The listing builds one solid part. Answer for the finished solid, in the listing's coordinates (mm). A direction names the side the tool comes from. Round coordinates to 2 decimals unless told otherwise and drop trailing zeros. Write each loop counter-clockwise with the first axis right and the second up, starting at its lowest first coordinate (ties: lowest second). Pieces come first, ordered by that corner, then holes. Notation, with made-up numbers: (67.25, -18) -> (97.25, -18) arc R16 ccw to (97.25, 9) -> close; hole circle Ø5 at (57, 84). An arc over 180 degrees is marked (long way). Write each question's results on one line, items separated by ' | '. Start each with the question number.
Autodesk Fusion 360 part; units mm, degrees
sketch "Sketch1" plane through (0, 0, 0) normal (0, 1, 0) x (1, 0, 0)
  line L0 (0, 0) -> (4, 0)
  line L1 (4, 0) -> (4, -4)
  line L2 (4, -4) -> (0, -4)
  line L3 (0, -4) -> (0, 0)
  circle A0 centre (2, -2) radius 0.8
  dimension "d1" = 4
  dimension "d2" = 4
  dimension "d3" = 1.6
  dimension "d4" = 2
  dimension "d5" = 2
extrude "Extrude1" add sketch "Sketch1" along normal blind 14 makes body 1
sketch "Sketch2" plane through (0, 0, 4) normal (0, 0, 1) x (-1, 0, 0)
  line L0 (0, 0) -> (-4, 0)
  line L1 (-4, 0) -> (-4, -14)
  line L2 (-4, -14) -> (0, -14)
  line L3 (0, -14) -> (0, 0)
  line L4 (-4, -14) -> (0, -14)
  line L5 (0, -14) -> (0, -10)
  line L6 (0, -10) -> (-4, -10)
  line L7 (-4, -10) -> (-4, -14)
  circle A0 centre (-2, -12) radius 0.8
  dimension "d8" = 4
  dimension "d9" = 1.6
  dimension "d10" = 2
  dimension "d11" = 2
extrude "Extrude2" add sketch "Sketch2" along normal blind 10 contours L1 L2 L3 L4 L5 L6 L7 bodies 1
ref_plane "WorkPlane1" through (4, 7, 0) normal (0.9397, 0, -0.342) x (0, 1, 0)
sketch "Sketch3" plane through (4, 7, 0) normal (0.9397, 0, -0.342) x (0, 1, 0)
  line L0 (-7, 3.7588) -> (-7, 0)
  line L1 (-7, 0) -> (7, 0)
  line L2 (7, 0) -> (7, 13.1557)
  line L3 (7, 13.1557) -> (3, 13.1557)
  line L4 (3, 13.1557) -> (3, 3.7588)
  line L5 (3, 3.7588) -> (-7, 3.7588)
  line L6 (7, 0) -> (3, 0)
  line L7 (3, 0) -> (3, 3.7588)
  line L8 (3, 3.7588) -> (7, 3.7588)
  line L9 (7, 3.7588) -> (7, 0)
  circle A0 centre (5, 1.7588) radius 0.8
  dimension "d15" = 1.6
  dimension "d16" = 2
  dimension "d17" = 2
extrude "Extrude3" add sketch "Sketch3" along normal blind 10 separate body contours L1 L2 L6 L7 L8 L9 makes body 2
extrude "Extrude4" add 1 faces at (5.1485, 12.0199, 3.1555) along direction (-0.939693, 0, 0.34202) up to surface end surface through (4, 0, 0) normal (1, 0, 0) offset 0 on bodies 2 bodies 2 1
extrude "Extrude5" add sketch "Sketch1" along normal blind 4 from surface at 10 contours A0 bodies 2
Q1. The part is cut by section B-B, the plane z = 8. Write down the section's boundary in (x, y).
Q2. Each of these flat-tipped pins is pushed along its axis until it touches: pin 1 (1.2 mm diameter, centred on y = 12.5, z = 11.5, fed in from +X); pin 2 (8 mm diameter, centred on x = 8, z = -0.5, fed in from -Y); pin 3 (4.5 mm diameter, centred on x = 1.5, y = 10.5, fed in from -Z); pin 4 (5 mm diameter, centred on x = 7, y = 3, fed in from -Z). Where does it stop, or does it pass through?
Q3. The part is cut by section A-A, the plane x = 2. Write down the section's boundary in (y, z).
Q4. Find the intervals of material crossed by line 1 (X direction, y = 12, z = 9.25); line 2 (Y direction, x = 2, z = 11.75), in increasing order.
Q5. Determine the mould class of faces 1 (the flat face through (2, 10, 9)), 2 (the flat face through (2, 12, 4)), 3 (the flat face through (2, 13, 14)) for opening direction Y: pulls with the +Y half, pulls with the -Y half, needs draft (parallel to the pull), parting line crosses it, or undercut.
Q6. The part is cut by section C-C, the plane y = 1.5. Write down the section's boundary in (x, z), then the cut area to 3 significant figures.
Q7. For faces 4 (the flat face through (9, 10, 0)), 5 (the flat face through (2, 10, 2)), 6 (the flat face through (2, 5, 4)), 7 (the flat face through (4, 12, 2)), determine the directions among +Z, -Z, +X, -X, +Y, -Y from which every point of the face is accessible in a straight line to the end or side of a thin tool.
Answers follow:
1) outline: (0, 10) -> (4, 10) -> (4, 14) -> (0, 14) -> close; hole circle Ø1.6 at (2, 12)
2) pin 1: x = 4 | pin 2: y = 10 | pin 3: z = 0 | pin 4: through
3) outline: (0, 0) -> (14, 0) -> (14, 14) -> (12.8, 14) -> (12.8, 4) -> (11.2, 4) -> (11.2, 14) -> (10, 14) -> (10, 4) -> (0, 4) -> (0, 2.8) -> (10, 2.8) -> (10, 1.2) -> (0, 1.2) -> close
4) line 1: 0 to 1.2, 2.8 to 4 | line 2: 10 to 11.2, 12.8 to 14
5) face 1: pulls with the -Y half | face 2: undercut | face 3: needs draft
6) outline: (0, 0) -> (4, 0) -> (4, 4) -> (0, 4) -> close; hole circle Ø1.6 at (2, 2) | area: 14.0 mm^2
7) face 4: +Z, -Z, +X, -Y | face 5: -Y | face 6: +Z, +X, -X, -Y | face 7: none
